Here's how the part is built. I have some questions about the finished solid (model axes, mm). Face numbers are marked on the shaded views. A direction names the side the tool comes from. Give positions to 0.01 mm unless a question says otherwise; leave off trailing zeros. Loops run counter-clockwise (first coordinate to the right, second up) from the corner with the lowest first, then second, coordinate; pieces in that order, holes last. Notation, with made-up numbers: (79, 22) - (115, 22) arc R33 cw to (115, 60) - close; hole circle Ø8 at (44, 66). An arc over 180 degrees is marked (long way). Put each result on its own line as item: value. Start each with the question number.
from build123d import *

# Parameters (mm, degrees)
BOSS_EXTRUDE1_DEPTH = 1.600000102
BOSS_EXTRUDE2_START = 1.6
BOSS_EXTRUDE2_DEPTH = 17.599999852
SKETCH7_W           = 6.999999716
SKETCH7_H           = 6.999999716
SKETCH7_W_2         = 9.650966474
SKETCH7_H_2         = 9.900528062
SKETCH7_H_3         = 10.408528062
SKETCH7_W_3         = 7.09362233
SKETCH7_H_4         = 7.09362233
BOSS_EXTRUDE4_DEPTH = 4.999999906
SKETCH2_R           = 1.5875
CUT_EXTRUDE3_DEPTH  = 107.667181296
SKETCH6_W           = 9.489999816
SKETCH6_H           = 12.599999946
SKETCH6_W_2         = 12.029999816
CUT_EXTRUDE1_DEPTH  = 7.64499995
FILLET1_R           = 2.000000064
CHAMFER2_SIZE       = 3
CUT_EXTRUDE6_DEPTH  = 2.50000008


with BuildPart() as part:
    # Sketch3 → Boss-Extrude1 (new body)
    with BuildSketch(Plane(origin=(0, 0, 0), x_dir=(1, 0, 0), z_dir=(0, 1, 0))):
        Polygon((72.079999858, 3.630252591), (80.996034335, 3.630252591), (80.996034335, -66.69999995), (-3.483453186, -66.69999995), (-3.483453186, -0.324999858), (-5.404999858, -0.324999858), (-5.404999858, 15.564999858), (-3.499999858, 15.564999858), (-3.499999858, 28.885000142), (-9.849999858, 28.885000142), (-9.849999858, 47.314999858), (-3.499999858, 47.314999858), (-3.499999858, 56.839999858), (65.965747409, 56.839999858), (69.539999858, 53.265747409), (69.539999858, 41.835747409), (72.079999858, 39.295747409), align=None)
    extrude(amount=BOSS_EXTRUDE1_DEPTH)

    # Sketch3<3> → Boss-Extrude2 (add)
    with BuildSketch(Plane(origin=(0, 0, 0), x_dir=(1, 0, 0), z_dir=(0, 1, 0)).offset(BOSS_EXTRUDE2_START)):
        Polygon((72.079999858, 3.630252591), (80.996034335, 3.630252591), (80.996034335, -66.69999995), (-3.483453186, -66.69999995), (-3.483453186, -0.324999858), (-5.404999858, -0.324999858), (-5.404999858, 15.564999858), (-3.499999858, 15.564999858), (-3.499999858, 28.885000142), (-9.849999858, 28.885000142), (-9.849999858, 47.314999858), (-3.499999858, 47.314999858), (-3.499999858, 56.839999858), (65.965747409, 56.839999858), (69.539999858, 53.265747409), (69.539999858, 41.835747409), (72.079999858, 39.295747409), align=None)
        Polygon((77.796034385, -0.705067354), (77.796034385, -63.5), (-0.299999908, -63.5), (-0.299999908, 0), (-0.299999908, 2.875000092), (-2.204999908, 2.875000092), (-2.204999908, 12.364999908), (-0.299999908, 12.364999908), (-0.299999908, 32.085000092), (-6.649999908, 32.085000092), (-6.649999908, 44.114999908), (-0.299999908, 44.114999908), (-0.299999908, 53.639999908), (64.640264031, 53.639999908), (66.339999908, 51.940264031), (66.339999908, 40.510264031), (68.879999908, 37.970264031), (68.879999908, 4.955735969), (66.339999908, 2.415735969), (66.339999908, 0), (66.339999908, -0.705067354), align=None, mode=Mode.SUBTRACT)
    extrude(amount=BOSS_EXTRUDE2_DEPTH)

    # Sketch7 → Boss-Extrude4 (add)
    with BuildSketch(Plane(origin=(0, 1.600000102, 0), x_dir=(1, 0, 0), z_dir=(0, 1, 0))):
        with Locations((15.24, 50.8)):
            Rectangle(SKETCH7_W, SKETCH7_H)
        with Locations((66.04, 35.56)):
            Rectangle(SKETCH7_W_2, SKETCH7_H_2)
        with Locations((66.04, 7.62)):
            Rectangle(SKETCH7_W_2, SKETCH7_H_3)
        with Locations((13.97, 2.54)):
            Rectangle(SKETCH7_W_3, SKETCH7_H_4)
    extrude(amount=BOSS_EXTRUDE4_DEPTH)

    # Sketch2 → Cut-Extrude3 (cut, through all)
    with BuildSketch(Plane(origin=(0, 0, 0), x_dir=(1, 0, 0), z_dir=(0, 1, 0))):
        with Locations(Location((13.97, 2.54, 0), (0, 0, 90))):
            Circle(SKETCH2_R)
        with Locations(Location((15.24, 50.8, 0), (0, 0, 270))):
            Circle(SKETCH2_R)
        with Locations(Location((66.04, 35.56, 0), (0, 0, 90))):
            Circle(SKETCH2_R)
        with Locations(Location((66.04, 7.62, 0), (0, 0, 270))):
            Circle(SKETCH2_R)
    extrude(amount=CUT_EXTRUDE3_DEPTH, mode=Mode.SUBTRACT)

    # Sketch6 → Cut-Extrude1 (cut)
    with BuildSketch(Plane(origin=(-2.204999908, 0, 0), x_dir=(0, 0, -1), z_dir=(1, 0, 0))):
        with Locations((7.62, 12.899999981)):
            Rectangle(SKETCH6_W, SKETCH6_H)
        with Locations((38.1, 12.899999981)):
            Rectangle(SKETCH6_W_2, SKETCH6_H)
    extrude(amount=-CUT_EXTRUDE1_DEPTH, mode=Mode.SUBTRACT)

    # Fillet1
    fillet1_edges = [part.edges().sort_by_distance(p)[0] for p in [
        (11.740000142, 4.100000055, -53.639999908),
        (18.739999858, 4.100000055, -53.639999908),
        (18.739999858, 4.100000055, -47.300000142),
        (11.740000142, 4.100000055, -47.300000142),
        (66.339999908, 4.100000004, -40.510264031),
        (68.879999908, 4.100000055, -30.609735969),
        (61.214516763, 4.100000055, -30.609735969),
        (61.214516763, 4.100000055, -40.510264031),
        (66.339999908, 4.100000004, -2.415735969),
        (68.879999908, 4.100000055, -12.824264031),
        (61.214516763, 4.100000055, -2.415735969),
        (61.214516763, 4.100000055, -12.824264031),
        (10.423188835, 4.100000055, -6.086811165),
        (10.423188835, 4.100000055, 1.006811165),
        (17.516811165, 4.100000055, 1.006811165),
        (17.516811165, 4.100000055, -6.086811165),
    ]]
    fillet(fillet1_edges, radius=FILLET1_R)

    # Chamfer2
    chamfer2_edges = [part.edges().sort_by_distance(p)[0] for p in [
        (-3.499999858, 9.599999926, -56.839999858),
        (80.996034335, 9.599999926, -3.630252591),
        (80.996034335, 9.599999926, 66.69999995),
        (-3.483453186, 9.599999926, 66.69999995),
        (-0.299999908, 10.399999926, 63.5),
        (77.796034385, 10.399999926, 63.5),
        (77.796034385, 10.399999926, 0.705067354),
    ]]
    chamfer(chamfer2_edges, length=CHAMFER2_SIZE)

    # Sketch15 → Cut-Extrude6 (cut)
    with BuildSketch(Plane.XZ):
        Polygon((13.97, 0.60655898), (11.244999989, -0.96672051), (11.244999989, -4.11327949), (13.97, -5.68655898), (16.695000011, -4.11327949), (16.695000011, -0.96672051), align=None)
        Polygon((66.04, -4.47344102), (63.314999989, -6.04672051), (63.314999989, -9.19327949), (66.04, -10.76655898), (68.765000011, -9.19327949), (68.765000011, -6.04672051), align=None)
        Polygon((66.04, -32.41344102), (63.314999989, -33.98672051), (63.314999989, -37.13327949), (66.04, -38.70655898), (68.765000011, -37.13327949), (68.765000011, -33.98672051), align=None)
        Polygon((15.24, -47.65344102), (12.514999989, -49.22672051), (12.514999989, -52.37327949), (15.24, -53.94655898), (17.965000011, -52.37327949), (17.965000011, -49.22672051), align=None)
    extrude(amount=-CUT_EXTRUDE6_DEPTH, mode=Mode.SUBTRACT)


solid = part.part
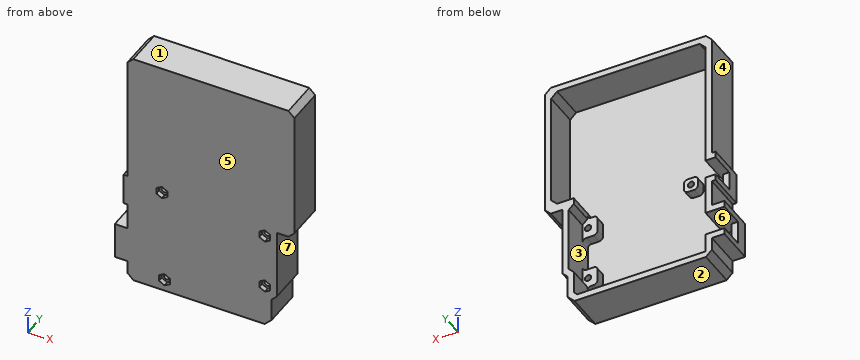
1) Which directions (+Z, -Z, +X, -X, +Y, -Y) give clear straight access to the entire face, cutting with the end or side of a thin tool? Please do the marked faces 5, 6 and 7.
2) Thinking about a two-plate mould opening in Z: for the marked faces 1, 2, 3 and 4, which applies, pulls with the +Z half, pulls with the -Z half, needs draft (parallel to the pull), parting line crosses it, or undercut?
3) Suppose I cut it at D-D on z = 24. Please give me the cut outline in (x, y).
4) Suppose I cut it at A-A on z = -7.62. Please give me the cut outline in (x, y) (1 decimal).
5) Suppose I cut it at B-B on y = 4.5. Give the number of separate pieces and of enclosed holes in the cut face, plus the area to 3 significant figures.
6) I'm going to push flat-ended pins straight in: P1, Ø1.8, axis at x = 76, y = 5.5, coming from the -Z side; P2, Ø7, axis at x = 15.5, z = -49, coming from the +Y side; P3, Ø6, axis at x = 60, z = -18, coming from the +Y side. Where does each tip first touch, or does it pass through?
7) Suppose I cut it at C-C on x = 26.5. Please give me the cut outline in (y, z).
8) I need wall thicknesses on line 1 (X direction, y = 3.6, z = -35.56); line 2 (X direction, y = 3.75, z = -7.62) (1 decimal); line 3 (Z direction, x = -2, y = 14.5) (3 decimals). Which ranges of each line are inside material? Lowest first, please.
Ans:
1. face 5: +Z, -Z, +X, -X, -Y
1. face 6: +Y
1. face 7: -Z, +X, +Y, -Y
2. face 1: pulls with the +Z half
2. face 2: pulls with the -Z half
2. face 3: undercut
2. face 4: needs draft
3. outline: (-3.48, 0) - (81, 0) - (81, 19.2) - (77.8, 19.2) - (77.8, 1.6) - (-0.3, 1.6) - (-0.3, 19.2) - (-3.48, 19.2) - close
4. outline: (-5.4, 0) - (63.3, 0) - (63.3, 2.5) - (64.5, 2.5) - (64.5, 6.6) - (61.2, 6.6) - (61.2, 1.6) - (-2.2, 1.6) - (-2.2, 6.6) - (-5.4, 6.6) - close; (67.6, 2.5) - (68.8, 2.5) - (68.8, 0) - (72.1, 0) - (72.1, 19.2) - (68.9, 19.2) - (68.9, 6.6) - (67.6, 6.6) - close
5. separate pieces: 2
5. enclosed holes: 5
5. area: 1,560 mm²
6. P1: stops at z = -3.63
6. P2: stops at y = 6.6
6. P3: stops at y = 1.6
7. outline: (0, -56.84) - (19.2, -56.84) - (19.2, -53.64) - (1.6, -53.64) - (1.6, 63.5) - (19.2, 63.5) - (19.2, 66.7) - (0, 66.7) - close
8. line 1: x = -9.85 to -6.65, 61.21 to 64.45, 67.63 to 72.08
8. line 2: x = -5.4 to -2.2, 61.2 to 64.5, 67.6 to 72.1
8. line 3: z = -55.34 to -44.115, -32.085 to -12.365, -2.875 to 65.183
